The drawing under review shows one solid part. Ordinate dimensions are in mm from its lowest x, y, z. A direction names the side the tool comes from. Give positions to 0.01 mm unless a question says otherwise; leave off trailing zeros. Order: outer loops, then holes, each group sorted by start corner. A loop starts at its lowest first (then second) coordinate and runs counter-clockwise, first axis right, second up. Notation, with made-up numbers: (18.25, 49) -> (71.25, 49) arc R4 ccw to (71.25, 54) -> close; hole circle Ø4 at (22, -28). An arc over 180 degrees is marked (long way). One line per item, written item: value. Start each with the question number.
1) Consider section B-B (x = 7.5). State the section outline as (y, z) points.
2) Wall thickness on line 1 along Z through (x, y) = (11.75, 3.25); line 2 along X through (y, z) = (4.5, 1.45); line 3 along Y through (x, z) = (8.75, 0.95): over which ranges is each line inside the solid? List them lowest first. Write a range as from..to.
3) For pin 1 (1.5 mm diameter, centred on x = 13, y = 1.5, fed in from -Z), flat-tipped, find the tip position at first contact; note if it passes through.
4) Tool access review of the marked faces 1 and 2: name each direction out of +Z, -Z, +X, -X, +Y, -Y from which nothing blocks a thin tool from reaching the whole face with its end or side.
5) Consider section A-A (y = 5). State the section outline as (x, z) points, plus the area to 3 significant figures.
6) Consider section D-D (x = 13.75). State the section outline as (y, z) points, plus the area to 3 significant figures.
7) Consider section C-C (z = 0.15). State the section outline as (x, y) points.
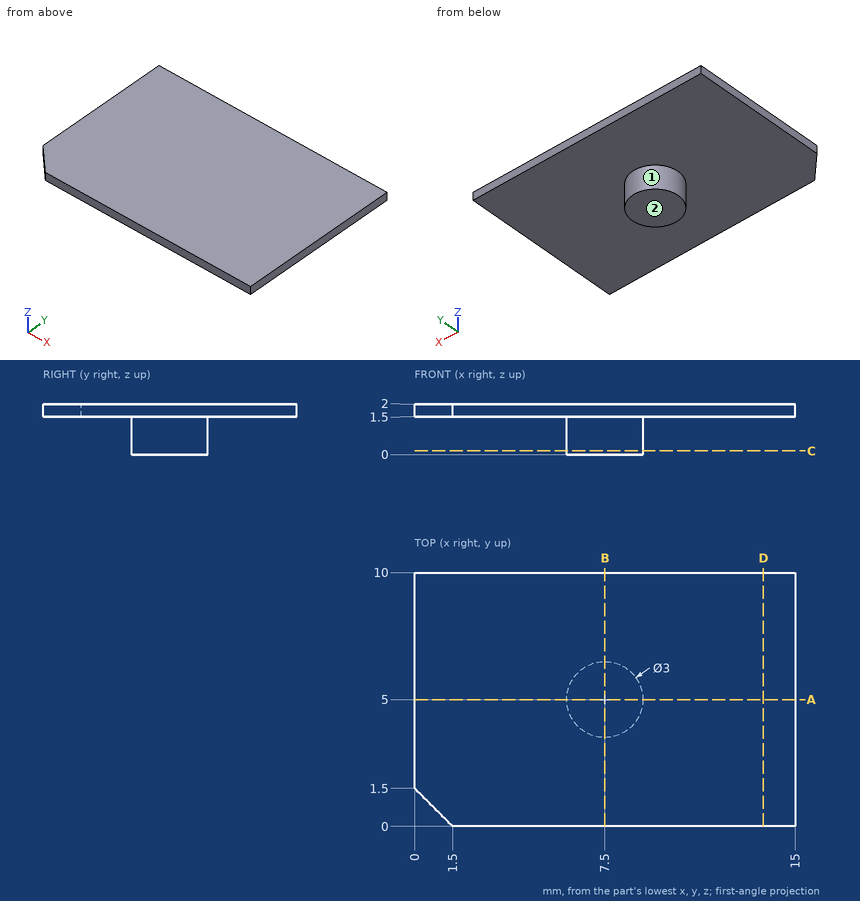
Checked values:
1. outline: (0, 1.5) -> (3.5, 1.5) -> (3.5, 0) -> (6.5, 0) -> (6.5, 1.5) -> (10, 1.5) -> (10, 2) -> (0, 2) -> close
2. line 1: z = 1.5..2
2. line 2: x = 6.09..8.91
2. line 3: y = 4.17..5.83
3. pin 1: stops at z = 1.5
4. face 1: -Z
4. face 2: -Z, +X, -X, +Y, -Y
5. outline: (0, 1.5) -> (6, 1.5) -> (6, 0) -> (9, 0) -> (9, 1.5) -> (15, 1.5) -> (15, 2) -> (0, 2) -> close
5. area: 12.0 mm^2
6. outline: (0, 1.5) -> (10, 1.5) -> (10, 2) -> (0, 2) -> close
6. area: 5.00 mm^2
7. outline: circle Ø3 at (7.5, 5)
